from build123d import *

# Parameters (mm, degrees)
M3X0_5_TAPPED_HOLE1_D      = 2.5
M3X0_5_TAPPED_HOLE1_DEPTH  = 7.5
M3X0_5_TAPPED_HOLE1_TIP    = 0.751075774
F_10_24_TAPPED_HOLE1_D     = 3.7973
F_10_24_TAPPED_HOLE1_DEPTH = 10
F_10_24_TAPPED_HOLE1_TIP   = 1.140824014


with BuildPart() as part:
    # Sketch1 → Revolve1 (revolve)
    with BuildSketch(Plane.XY):
        Polygon((0, 13.8025), (6.5, 13.8025), (6.5, 4.8), (7.5, 4.8), (7.5, 0), (0, 0), align=None)
    revolve(axis=Axis((0, 0, 0), (0, 1, 0)))

    # M3x0.5 Tapped Hole1
    with Locations(Plane(origin=(0, 0, 0), x_dir=(-1, 0, 0), z_dir=(0, -1, 0))):
        with Locations((0, 5), (4.330127019, -2.5), (-4.330127019, -2.5)):
            Hole(M3X0_5_TAPPED_HOLE1_D / 2, depth=M3X0_5_TAPPED_HOLE1_DEPTH)
            with Locations((0, 0, -(M3X0_5_TAPPED_HOLE1_DEPTH + M3X0_5_TAPPED_HOLE1_TIP / 2))):  # 118° drill point
                Cone(0, M3X0_5_TAPPED_HOLE1_D / 2, M3X0_5_TAPPED_HOLE1_TIP, mode=Mode.SUBTRACT)

    # #10-24 Tapped Hole1
    with Locations(Plane(origin=(0, 13.8025, 0), x_dir=(1, 0, 0), z_dir=(0, 1, 0))):
        with Locations((0, 0)):
            Hole(F_10_24_TAPPED_HOLE1_D / 2, depth=F_10_24_TAPPED_HOLE1_DEPTH)
            with Locations((0, 0, -(F_10_24_TAPPED_HOLE1_DEPTH + F_10_24_TAPPED_HOLE1_TIP / 2))):  # 118° drill point
                Cone(0, F_10_24_TAPPED_HOLE1_D / 2, F_10_24_TAPPED_HOLE1_TIP, mode=Mode.SUBTRACT)


solid = part.part
Could you check a few things on this model? Use its own coordinates, in mm. A direction names the side the tool comes from. Round coordinates to 2 decimals unless told otherwise and drop trailing zeros. Write each loop counter-clockwise with the first axis right and the second up, starting at its lowest first coordinate (ties: lowest second). Pieces come first, ordered by that corner, then holes. Notation, with made-up numbers: (15, 14.25) - (40, 14.25) arc R11 ccw to (40, 22.25) - close; hole circle Ø5 at (32, -31). An arc over 180 degrees is marked (long way). Put each result on its own line as item: value. Start each with the question number.
(1) I want a section at A-A, the plane y = 9.75. Please give me the cut outline in (x, z), plus the area to 3 significant figures.
(2) I need wall thicknesses on probe 1 along Z at (x, y) = (0, 6.5); probe 2 along Z at (x, y) = (0, 8.5); probe 3 along Z at (x, y) = (-0.5, 5.75). Which ranges of each line are inside material? Lowest first, please.
(3) Thinking about a two-plate mould opening in Z: for faces 1 (the cylindrical face through (5.52, 3.8, 2.12)), 2 (the cylindrical face through (-5.158, 9.238, 3.955)), 3 (the flat face through (-1, 13.802, -2)), which applies, released by +Z, released by -Z, zero draft, split by the parting line, or undercut?
(4) I want a section at C-C, the plane y = 7.75. Please give me the cut outline in (x, z).
(5) I want a section at B-B, the plane z = -2.25. Please give me the cut outline in (x, y), plus the area to 3 significant figures.
(6) For faces 4 (the cylindrical face through (-0.27, 3.8, -3.78)), 5 (the flat face through (6, 4.8, -3)), 6 (the cylindrical face through (-7.493, 2.366, -0.33)), which set-ups out of +Z, -Z, +X, -X, +Y, -Y let a thin tool reach every point of the face, with its end or its side?
(7) Will these pins go through, and if not, where does the flat tip stop? pin 1 (1 mm diameter, centred on y = 10, z = 4, fed in from -X); pin 2 (2 mm diameter, centred on x = -4.33, z = 2.5, fed in from -Y); pin 3 (6 mm diameter, centred on x = 4, y = 7.5, fed in from +Z); pin 4 (6 mm diameter, centred on x = -2.5, y = 6.5, fed in from +Z).
Here are the results:
1. outline: circle Ø13 at (0, 0); hole circle Ø3.8 at (0, 0)
1. area: 121 mm^2
2. probe 1: z = -6.5 to -6.25, -3.75 to -1.9, 1.9 to 6.5
2. probe 2: z = -6.5 to -1.9, 1.9 to 6.5
2. probe 3: z = -6.48 to -6.15, -3.85 to -1.83, 1.83 to 6.48
3. face 1: undercut
3. face 2: split by the parting line
3. face 3: zero draft
4. outline: circle Ø13 at (0, 0); hole circle Ø1.67 at (-4.33, 2.5); hole circle Ø3.8 at (0, 0); hole circle Ø1.67 at (0, -5); hole circle Ø1.67 at (4.33, 2.5)
5. outline: (-7.15, 0) - (7.15, 0) - (7.15, 4.8) - (6.1, 4.8) - (6.1, 13.8) - (-6.1, 13.8) - (-6.1, 4.8) - (-7.15, 4.8) - close
5. area: 178 mm^2
6. face 4: -Y
6. face 5: +Y
6. face 6: +Y, -Y
7. pin 1: stops at x = -5.48
7. pin 2: stops at y = 7.65
7. pin 3: stops at z = 7
7. pin 4: stops at z = 7.5
